Could you check a few things on this model? Use its own coordinates, in mm. A direction names the side the tool comes from. Round coordinates to 2 decimals unless told otherwise and drop trailing zeros. Write each loop counter-clockwise with the first axis right and the second up, starting at its lowest first coordinate (ties: lowest second). Pieces come first, ordered by that corner, then holes. Notation, with made-up numbers: (29, -3) -> (47, -3) arc R13 ccw to (47, 18) -> close; hole circle Ø10 at (37.5, 78.5). An arc over 180 degrees is marked (long way). One line per question, with ' | ' between items. Start each with the question number.
1. Imagine slicing it at B-B, the plane x = 156.25. List the corners of the cut face in (y, z) for me, and give its area (3 significant figures).
2. Imagine slicing it at A-A, the plane y = 6.25. List the corners of the cut face in (x, z) for me, and give its area (3 significant figures).
3. For faces 1 (the flat face through (130.7, 16.8, -162.8)), 2 (the flat face through (19, 18, -160)), 3 (the cylindrical face through (16.7, 16.48, -32.07)), 4 (the flat face through (23.199, 16.479, -155.995)), 5 (the cylindrical face through (32.47, 15.59, -167.39)), which set-ups out of +Z, -Z, +X, -X, +Y, -Y let a thin tool reach every point of the face, with its end or its side?
4. Thinking about a two-plate mould opening in Z: for faces 6 (the flat face through (230, 10, -175.35)), 7 (the flat face through (117, 0, -174)), 8 (the flat face through (11.69, 16.8, -27.77)), which applies, released by +Z, released by -Z, zero draft, split by the parting line, or undercut?
5. Imagine slicing it at C-C, the plane z = -77. List the corners of the cut face in (x, y) for me, and give its area (3 significant figures).
6. For pin 1 Ø3.5 at (x, z) = (133.5, -163) entering from +Y; pin 2 Ø8 at (x, z) = (132.25, -163.5) entering from -Y; pin 3 Ø5.5 at (x, z) = (29, -167.85) entering from -Y, each with a flat end and sliding along its axis, tell me the tip position at first contact or that it passes through.
7. If I drill on line 1 along X through (y, z) = (16.4, -163.5) (3 decimals); line 2 along X through (y, z) = (17.7, -163.5) (3 decimals); line 3 along X through (y, z) = (17.25, -24.8) (3 decimals), over which ranges is the centre line in solid material (lowest first)? Write a range as [from, to].
8. Imagine slicing it at D-D, the plane x = 64. List the corners of the cut face in (y, z) for me.
from build123d import *

# Parameters (mm, degrees)
EXTRUDE_1_DEPTH     = 20
EXTRUDE_START       = 1
SKETCH_2_R          = 1.525
EXTRUDE_2_DEPTH     = 3
CUT_EXTRUDE_1_REACH = 358.708
SKETCH_3_W          = 31
SKETCH_3_H          = 9.5
SKETCH_4_R          = 3.5
CUT_EXTRUDE_2_DEPTH = 1.2
CUT_EXTRUDE_3_REACH = 356.959
SKETCH_5_R          = 1.525
FILLET_1_R          = 1
FILLET_3_R          = 1
SKETCH_6_R          = 3.5
CUT_EXTRUDE_4_DEPTH = 1.2
SKETCH_7_W          = 69.4
SKETCH_7_H          = 20
CUT_EXTRUDE_5_DEPTH = 3
SKETCH_8_W          = 20
SKETCH_8_H          = 20
CUT_EXTRUDE_6_DEPTH = 1.5
FILLET_4_R          = 2
FILLET_5_R          = 2
FILLET_6_R          = 2
CUT_EXTRUDE_7_DEPTH = 10
FILLET_7_R          = 1
FILLET_8_R          = 1


with BuildPart() as part:
    # 草图1 → 凸台-拉伸1 (new body)
    with BuildSketch(Plane(origin=(0, 0, 0), x_dir=(1, 0, 0), z_dir=(0, 1, 0))):
        Polygon((1.5, 0), (3, 0), (3, 173.85), (307.4, 173.85), (307.4, 176.85), (0, 176.85), (0, 0), (0, -3), (1.5, -3), align=None)
    extrude(amount=EXTRUDE_1_DEPTH)

    # 草图2 → 凸台-拉伸2 (add)
    # profile 1 of 3: a face of its own
    with BuildSketch(Plane(origin=(0, 14, 0), x_dir=(1, 0, 0), z_dir=(0, 1, 0)).offset(EXTRUDE_START)):
        Polygon((3, 153.85), (25, 173.85), (42.839282497, 173.85), (3, 137.632470457), align=None)
        with Locations(Location((20.25, 163.5, 0), (0, 0, 270))):
            Circle(SKETCH_2_R, mode=Mode.SUBTRACT)
    # profile 2 of 3: a face of its own
    with BuildSketch(Plane(origin=(0, 14, 0), x_dir=(1, 0, 0), z_dir=(0, 1, 0)).offset(EXTRUDE_START)):
        with BuildLine():
            Line((137.25, 163.5), (137.25, 173.85))
            Line((137.25, 173.85), (127.25, 173.85))
            Line((127.25, 173.85), (127.25, 163.5))
            ThreePointArc((127.25, 163.5), (132.25, 158.5), (137.25, 163.5))
        make_face()
        with Locations(Location((132.25, 163.5, 0), (0, 0, 270))):
            Circle(SKETCH_2_R, mode=Mode.SUBTRACT)
    # profile 3 of 3: a face of its own
    with BuildSketch(Plane(origin=(0, 14, 0), x_dir=(1, 0, 0), z_dir=(0, 1, 0)).offset(EXTRUDE_START)):
        with BuildLine():
            Line((3, 23.870342351), (3, 33.5))
            Line((3, 33.5), (13.2, 33.5))
            ThreePointArc((13.2, 33.5), (16.735533906, 32.035533906), (18.2, 28.5))
            Line((18.2, 28.5), (18.2, 15.043961292))
            Line((18.2, 15.043961292), (3, 15.043961292))
            Line((3, 15.043961292), (3, 23.870342351))
        make_face()
        with Locations(Location((13.2, 28.5, 0), (0, 0, 270))):
            Circle(SKETCH_2_R, mode=Mode.SUBTRACT)
    extrude(amount=EXTRUDE_2_DEPTH)

    # 草图3 → 切除-拉伸1 (cut, up to next)
    with BuildSketch(Plane(origin=(0, 0, -176.85), x_dir=(-1, 0, 0), z_dir=(0, 0, -1)), mode=Mode.PRIVATE) as cut_extrude_1_sk1:
        with Locations((-291.9, 15.25)):
            Rectangle(SKETCH_3_W, SKETCH_3_H)
    cut_extrude_1_tool1 = extrude(cut_extrude_1_sk1.sketch, amount=-CUT_EXTRUDE_1_REACH, mode=Mode.PRIVATE) & part.part
    add(cut_extrude_1_tool1.solids().sort_by_distance((291.9, 15.25, -176.85))[0], mode=Mode.SUBTRACT)

    # 草图4 → 切除-拉伸2 (cut)
    with BuildSketch(Plane(origin=(0, 18, 0), x_dir=(1, 0, 0), z_dir=(0, 1, 0))):
        with Locations(Location((13.2, 28.5, 0), (0, 0, 270))):
            Circle(SKETCH_4_R)
        with Locations(Location((20.25, 163.5, 0), (0, 0, 270))):
            Circle(SKETCH_4_R)
        with Locations(Location((132.25, 163.5, 0), (0, 0, 270))):
            Circle(SKETCH_4_R)
    extrude(amount=-CUT_EXTRUDE_2_DEPTH, mode=Mode.SUBTRACT)

    # 草图5 → 切除-拉伸3 (cut, up to next)
    with BuildSketch(Plane.XZ.offset(-15), mode=Mode.PRIVATE) as cut_extrude_3_sk1:
        with Locations(Location((29, -167.85, 0), (0, 0, 270))):
            Circle(SKETCH_5_R)
    cut_extrude_3_tool1 = extrude(cut_extrude_3_sk1.sketch, amount=-CUT_EXTRUDE_3_REACH, mode=Mode.PRIVATE) & part.part
    # 草图5 → 切除-拉伸3 (cut, up to next)
    with BuildSketch(Plane.XZ.offset(-15), mode=Mode.PRIVATE) as cut_extrude_3_sk2:
        with Locations(Location((8, -150.85, 0), (0, 0, 270))):
            Circle(SKETCH_5_R)
    cut_extrude_3_tool2 = extrude(cut_extrude_3_sk2.sketch, amount=-CUT_EXTRUDE_3_REACH, mode=Mode.PRIVATE) & part.part
    # 草图5 → 切除-拉伸3 (cut, up to next)
    with BuildSketch(Plane.XZ.offset(-15), mode=Mode.PRIVATE) as cut_extrude_3_sk3:
        with Locations(Location((8, -24.8, 0), (0, 0, 270))):
            Circle(SKETCH_5_R)
    cut_extrude_3_tool3 = extrude(cut_extrude_3_sk3.sketch, amount=-CUT_EXTRUDE_3_REACH, mode=Mode.PRIVATE) & part.part
    add(cut_extrude_3_tool1.solids().sort_by_distance((29, 15, -167.85))[0], mode=Mode.SUBTRACT)
    add(cut_extrude_3_tool2.solids().sort_by_distance((8, 15, -150.85))[0], mode=Mode.SUBTRACT)
    add(cut_extrude_3_tool3.solids().sort_by_distance((8, 15, -24.8))[0], mode=Mode.SUBTRACT)

    # 圆角1
    fillet_1_edges = [part.edges().sort_by_distance(p)[0] for p in [
        (0, 10, -176.85),
    ]]
    fillet(fillet_1_edges, radius=FILLET_1_R)

    # 圆角3
    fillet_3_edges = [part.edges().sort_by_distance(p)[0] for p in [
        (276.4, 10.5, -175.35),
    ]]
    fillet(fillet_3_edges, radius=FILLET_3_R)

    # 草图6 → 切除-拉伸4 (cut)
    with BuildSketch(Plane.XZ.offset(-15)):
        with Locations(Location((8, -24.8, 0), (0, 0, 270))):
            Circle(SKETCH_6_R)
        with Locations(Location((8, -150.85, 0), (0, 0, 270))):
            Circle(SKETCH_6_R)
        with Locations(Location((29, -167.85, 0), (0, 0, 270))):
            Circle(SKETCH_6_R)
    extrude(amount=-CUT_EXTRUDE_4_DEPTH, mode=Mode.SUBTRACT)

    # 草图7 → 切除-拉伸5 (cut)
    with BuildSketch(Plane(origin=(0, 0, -176.85), x_dir=(-1, 0, 0), z_dir=(0, 0, -1))):
        with Locations((-272.7, 10)):
            Rectangle(SKETCH_7_W, SKETCH_7_H)
    extrude(amount=-CUT_EXTRUDE_5_DEPTH, mode=Mode.SUBTRACT)

    # 草图8 → 切除-拉伸6 (cut)
    with BuildSketch(Plane(origin=(0, 0, -176.85), x_dir=(-1, 0, 0), z_dir=(0, 0, -1))):
        with Locations((-228, 10)):
            Rectangle(SKETCH_8_W, SKETCH_8_H)
    extrude(amount=-CUT_EXTRUDE_6_DEPTH, mode=Mode.SUBTRACT)

    # 圆角4
    fillet_4_edges = [part.edges().sort_by_distance(p)[0] for p in [
        (218, 20, -176.1),
        (218, 0, -176.1),
    ]]
    fillet(fillet_4_edges, radius=FILLET_4_R)

    # 圆角5
    fillet_5_edges = [part.edges().sort_by_distance(p)[0] for p in [
        (238, 20, -174.6),
        (238, 0, -174.6),
    ]]
    fillet(fillet_5_edges, radius=FILLET_5_R)

    # 圆角6
    fillet_6_edges = [part.edges().sort_by_distance(p)[0] for p in [
        (18.2, 16.5, -15.043961292),
    ]]
    fillet(fillet_6_edges, radius=FILLET_6_R)

    # 草图9 → 切除-拉伸7 (cut)
    with BuildSketch(Plane.XY.offset(-173.85)):
        with BuildLine():
            Line((152.25, 15), (152.25, 20))
            Line((152.25, 20), (160.25, 20))
            Line((160.25, 20), (160.25, 15))
            ThreePointArc((160.25, 15), (156.25, 11), (152.25, 15))
        make_face()
        with BuildLine():
            Line((168.25, 15), (168.25, 20))
            Line((168.25, 20), (176.25, 20))
            Line((176.25, 20), (176.25, 15))
            ThreePointArc((176.25, 15), (172.25, 11), (168.25, 15))
        make_face()
    extrude(amount=-CUT_EXTRUDE_7_DEPTH, mode=Mode.SUBTRACT)

    # 圆角7
    fillet_7_edges = [part.edges().sort_by_distance(p)[0] for p in [
        (156.25, 11, -176.85),
        (152.25, 17.5, -176.85),
        (160.25, 17.5, -176.85),
    ]]
    fillet(fillet_7_edges, radius=FILLET_7_R)

    # 圆角8
    fillet_8_edges = [part.edges().sort_by_distance(p)[0] for p in [
        (172.25, 11, -176.85),
        (168.25, 17.5, -176.85),
        (176.25, 17.5, -176.85),
    ]]
    fillet(fillet_8_edges, radius=FILLET_8_R)


solid = part.part
Geometry results:
1) outline: (0, -176.85) -> (10, -176.85) arc R1 ccw to (11, -175.85) -> (11, -173.85) -> (0, -173.85) -> close | area: 32.8 mm2
2) outline: (0, -175.85) arc R1 ccw to (1, -176.85) -> (218, -176.85) -> (218, -175.35) -> (238, -175.35) -> (238, -173.85) -> (3, -173.85) -> (3, 0) -> (1.5, 0) -> (1.5, 3) -> (0, 3) -> close | area: 1,210 mm2
3) face 1: +Y | face 2: +Z, +X, +Y | face 3: +X, +Y, -Y | face 4: +Y, -Y | face 5: -Y
4) face 6: released by -Z | face 7: zero draft | face 8: undercut
5) outline: (0, 0) -> (3, 0) -> (3, 20) -> (0, 20) -> close | area: 60.0 mm2
6) pin 1: stops at y = 16.8 | pin 2: stops at y = 15 | pin 3: stops at y = 16.2
7) line 1: x = [0, 3], [13.615, 18.725], [21.775, 31.454], [127.25, 130.725], [133.775, 137.25] | line 2: x = [0, 3], [13.615, 16.75], [23.75, 31.454], [127.25, 128.75], [135.75, 137.25] | line 3: x = [0, 6.475], [9.525, 18.2]
8) outline: (0, -176.85) -> (20, -176.85) -> (20, -173.85) -> (0, -173.85) -> close
